Geometry check sheet. Reference: drawing and pictorial views, mm from the part's lowest x, y, z. A direction names the side the tool comes from. Give positions to 0.01 mm unless a question says otherwise; leave off trailing zeros. Order: outer loops, then holes, each group sorted by start corner. A loop starts at its lowest first (then second) coordinate and runs counter-clockwise, first axis right, second up.
Item 1: Sectioned sample at B-B on x = 2. Record the boundary of the cut face in (y, z).
Item 2: Material ranges on line 1 along Y through (x, z) = (1.25, 56.3); line 2 along Y through (x, z) = (14, 43.7); line 3 along Y through (x, z) = (22.1, 21.15), recorded low to high.
Item 3: Release check for a two-part mould opening along Z. For the marked faces 5, 6 and 7 record: released by +Z, released by -Z, zero draft, split by the parting line, or undercut.
Item 4: Gauge pin test, flat ends, axial feed: P1, Ø1.5, axis at x = 4, y = 15, coming from the -Z side; P2, Ø6, axis at y = 38, z = 56, coming from the +X side; P3, Ø4.5, axis at y = 11.5, z = 44, coming from the -X side. Record the tip position at first contact, or that the pin passes through.
Item 5: Sectioned sample at C-C on x = 22.25. Record the boundary of the cut face in (y, z), and give its area (3 significant figures).
Item 6: Access from +Z, -Z, +X, -X, +Y, -Y to the whole of each face (thin tool, end or side, straight path). Record for the marked faces 1, 2, 3 and 4.
Item 7: Sectioned sample at D-D on y = 59.5. Record the boundary of the cut face in (x, z), and give its area (3 significant figures).
Item 8: Sectioned sample at A-A on z = 56.3. Record the boundary of the cut face in (x, y), and give its area (3 significant figures).
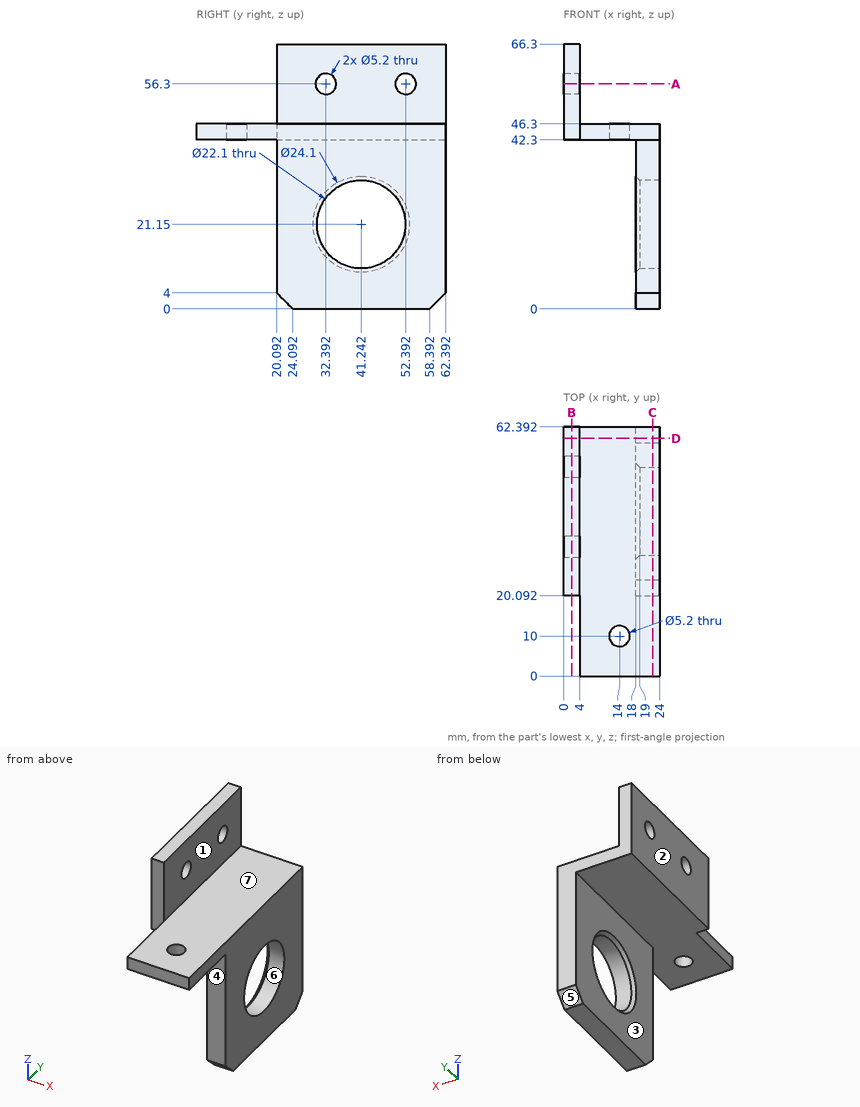
Report:
1. outline: (20.09, 42.3) - (62.39, 42.3) - (62.39, 66.3) - (20.09, 66.3) - close; hole circle Ø5.2 at (32.39, 56.3); hole circle Ø5.2 at (52.39, 56.3)
2. line 1: y = 20.09 to 29.79, 34.99 to 49.79, 54.99 to 62.39
2. line 2: y = 0 to 7.4, 12.6 to 62.39
2. line 3: y = 20.09 to 30.19, 52.29 to 62.39
3. face 5: released by -Z
3. face 6: undercut
3. face 7: released by +Z
4. P1: stops at z = 42.3
4. P2: stops at x = 4
4. P3: stops at x = 4
5. outline: (0, 42.3) - (20.09, 42.3) - (20.09, 4) - (24.09, 0) - (58.39, 0) - (62.39, 4) - (62.39, 46.3) - (0, 46.3) - close; hole circle Ø22.1 at (41.24, 21.15)
5. area: 1,640 mm2
6. face 1: +Z, +X, +Y, -Y
6. face 2: +Z, -Z, -X, +Y, -Y
6. face 3: -Z, -X, +Y, -Y
6. face 4: -Z, +X, -X, -Y
7. outline: (0, 42.3) - (18, 42.3) - (18, 1.11) - (24, 1.11) - (24, 46.3) - (4, 46.3) - (4, 66.3) - (0, 66.3) - close
7. area: 423 mm2
8. outline: (0, 20.09) - (4, 20.09) - (4, 29.79) - (0, 29.79) - close; (0, 34.99) - (4, 34.99) - (4, 49.79) - (0, 49.79) - close; (0, 54.99) - (4, 54.99) - (4, 62.39) - (0, 62.39) - close
8. area: 128 mm2
